Could you check a few things on this model? Use its own coordinates, in mm. A direction names the side the tool comes from. Coordinates: 2 decimals unless noted, no trailing zeros. Order: outer loops, then holes, each group sorted by start corner. A loop starts at its lowest first (then second) coordinate and runs counter-clockwise, first axis right, second up. Notation, with made-up numbers: (9, 15.25) - (16, 15.25) arc R34 cw to (16, 45.25) - close; hole circle Ø11 at (68.5, -18). An arc over 180 degrees is marked (long way). Answer as CSV lines item,"result". Start each with the question number.
1. Thinking about a two-plate mould opening in Z: for faces 3 (the face through (-94, 3, 86.444)), 4 (the face through (-131.445, 3, -109)), 5 (the face through (-94, 3, -86.444)), 6 (the face through (-2, 3, 131.7)), which applies, released by +Z, released by -Z, zero draft, split by the parting line, or undercut?
2. I want a section at C-C, the plane y = 3.75. Count the separate pieces of the cut face and the enclosed holes in it, and give its area (3 significant figures).
3. I want a section at A-A, the plane x = 11. List the corners of the cut face in (y, z) for me, and give its area (3 significant figures).
4. I need wall thicknesses on probe 1 along Z at (x, y) = (109, 2.75); probe 2 along Z at (x, y) = (29, 3.75); probe 3 along Z at (x, y) = (-85.5, 2.25). Which ranges of each line are inside material? Lowest first, please.
5. I want a section at D-D, the plane z = 78. List the corners of the cut face in (x, y) for me (3 decimals), and give its area (3 significant figures).
6. I want a section at B-B, the plane z = 14. List the corners of the cut face in (x, y) for me (3 decimals).
7. For faces 1 (the face through (-55.245, 3, 1)), 2 (the face through (-31.1, 6.35, -1.8)), which set-ups out of +Z, -Z, +X, -X, +Y, -Y let a thin tool reach every point of the face, with its end or its side?
from build123d import *

# Parameters (mm, degrees)
SKETCH1_W             = 262.89
SKETCH1_H             = 263.40054
SKETCH1_R             = 62.6745
BOSS_EXTRUDE1_DEPTH   = 6.35
F_6_CLEARANCE_HOLE1_D = 3.7973
F_6_CLEARANCE_HOLE2_D = 3.7973
F_6_CLEARANCE_HOLE3_D = 3.7973
SKETCH9_W             = 76.2
SKETCH9_H             = 172.887951896
CUT_EXTRUDE1_DEPTH    = 7.62


with BuildPart() as part:
    # Sketch1 → Boss-Extrude1 (new body)
    with BuildSketch(Plane(origin=(0, 0, 0), x_dir=(1, 0, 0), z_dir=(0, 1, 0))):
        Rectangle(SKETCH1_W, SKETCH1_H)
        with Locations(Location((31.75, 0, 0), (0, 0, 270))):
            Circle(SKETCH1_R, mode=Mode.SUBTRACT)
    extrude(amount=BOSS_EXTRUDE1_DEPTH)

    # #6 Clearance Hole1 (through all)
    with Locations(Plane(origin=(0, 6.35, 0), x_dir=(1, 0, 0), z_dir=(0, 1, 0))):
        with Locations((31.75, 66.94678), (-35.19678, 0), (98.69678, 0), (31.75, -66.94678)):
            Hole(F_6_CLEARANCE_HOLE1_D / 2)

    # #6 Clearance Hole2 (through all)
    with Locations(Plane(origin=(0, 6.35, 0), x_dir=(1, 0, 0), z_dir=(0, 1, 0))):
        with Locations((121.285, -121.54027), (108.585, -121.54027), (78.105, -121.54027), (65.405, -121.54027)):
            f_6_clearance_hole2 = Hole(F_6_CLEARANCE_HOLE2_D / 2)

    # Mirror1: #6 Clearance Hole2 across plane
    add(f_6_clearance_hole2.mirror(Plane.XY), mode=Mode.SUBTRACT)

    # #6 Clearance Hole3 (through all)
    with Locations(Plane(origin=(0, 6.35, 0), x_dir=(1, 0, 0), z_dir=(0, 1, 0))):
        with Locations((-43.815, -121.54027), (-56.515, -121.54027), (-86.995, -121.54027), (-99.695, -121.54027)):
            f_6_clearance_hole3 = Hole(F_6_CLEARANCE_HOLE3_D / 2)

    # Mirror2: #6 Clearance Hole3 across plane
    add(f_6_clearance_hole3.mirror(Plane.XY), mode=Mode.SUBTRACT)

    # Sketch9 → Cut-Extrude1 (cut)
    with BuildSketch(Plane(origin=(0, 6.35, 0), x_dir=(1, 0, 0), z_dir=(0, 1, 0))):
        with Locations((-93.345, 0)):
            Rectangle(SKETCH9_W, SKETCH9_H)
    extrude(amount=-CUT_EXTRUDE1_DEPTH, mode=Mode.SUBTRACT)


solid = part.part
Solved:
1,face 3,"undercut"
1,face 4,"zero draft"
1,face 5,"undercut"
1,face 6,"released by +Z"
2,separate pieces,"1"
2,enclosed holes,"21"
2,area,"43,500 mm2"
3,outline,"(0, -131.7) - (6.35, -131.7) - (6.35, -59.14) - (0, -59.14) - close; (0, 59.14) - (6.35, 59.14) - (6.35, 131.7) - (0, 131.7) - close"
3,area,"922 mm2"
4,probe 1,"z = -131.7 to -123.39, -119.69 to 119.69, 123.39 to 131.7"
4,probe 2,"z = -131.7 to -62.61, 62.61 to 131.7"
4,probe 3,"z = -131.7 to -122.71, -120.37 to -86.44, 86.44 to 120.37, 122.71 to 131.7"
5,outline,"(-55.245, 0) - (131.445, 0) - (131.445, 6.35) - (-55.245, 6.35) - close"
5,area,"1,190 mm2"
6,outline,"(-55.245, 0) - (-29.341, 0) - (-29.341, 6.35) - (-55.245, 6.35) - close; (92.841, 0) - (131.445, 0) - (131.445, 6.35) - (92.841, 6.35) - close"
7,face 1,"-X, +Y, -Y"
7,face 2,"+Z, -Z, +X, -X, +Y"
